from build123d import *

# Parameters (mm, degrees)
F2_SIZE2 = 1.8330871047
F2_SIZE  = 3.175
F3_R     = 0.762
F4_R     = 0.254
F5_SIZE  = 0.508
F6_R     = 2.0447
F7_DEPTH = 25.4


with BuildPart() as f1:
    # F0 (on Front) → F1 (revolve)
    with BuildSketch(Plane.XZ):
        Polygon((11.1125, 23.68296), (11.1125, 31.75), (0, 31.75), (0, 17.3101), (33.3375, 17.3101), (33.3375, 23.68296), (25.5905, 23.68296), (25.5905, 19.09445), (18.3261, 19.09445), (18.3261, 23.68296), align=None)
    revolve(axis=Axis((23.780265148, 0, 0), (1, 0, 0)))

    # F2
    f2_edges = [f1.edges().sort_by_distance(p)[0] for p in [
        (33.3375, 0, -23.68296),
    ]]
    f2_side = f1.faces().sort_by_distance((29.464, 0, -23.68296))[0]
    chamfer(f2_edges, length=F2_SIZE, length2=F2_SIZE2, reference=f2_side)

    # F3
    f3_edges = [f1.edges().sort_by_distance(p)[0] for p in [
        (18.3261, 0, -19.09445),
        (25.5905, 0, -19.09445),
    ]]
    fillet(f3_edges, radius=F3_R)

    # F4
    f4_edges = [f1.edges().sort_by_distance(p)[0] for p in [
        (11.1125, 0, -23.68296),
    ]]
    fillet(f4_edges, radius=F4_R)

    # F5
    f5_edges = [f1.edges().sort_by_distance(p)[0] for p in [
        (11.1125, 0, -31.75),
        (0, 0, -31.75),
    ]]
    chamfer(f5_edges, length=F5_SIZE)

    # F6 (on Right) → F7 (cut)
    with BuildSketch(Plane.YZ):
        with Locations((0, 26.9875)):
            Circle(F6_R)
        with Locations((23.3718605846, -13.49375)):
            Circle(F6_R)
        with Locations((-23.3718605846, -13.49375)):
            Circle(F6_R)
    extrude(amount=F7_DEPTH, mode=Mode.SUBTRACT)


solid = f1.part
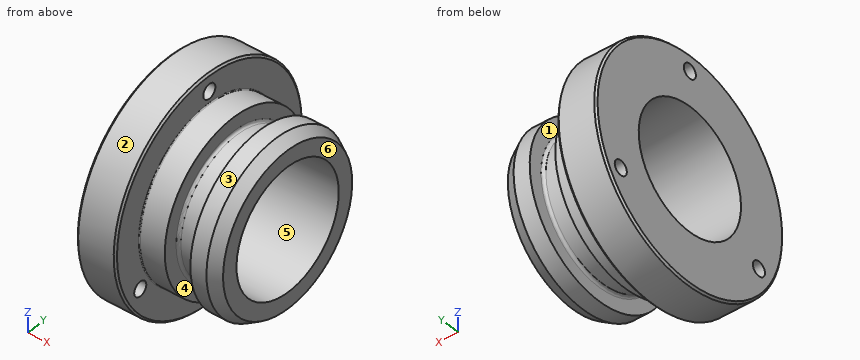
Input: part model. Units: mm. Frame: model coordinates. Face numbers are marked on the shaded views. A direction names the side the tool comes from. Coordinates: 2 decimals unless noted, no trailing zeros. Write each loop counter-clockwise with the first axis right and the second up, starting at its lowest first coordinate (ties: lowest second). Pieces come first, ordered by that corner, then holes. Notation, with made-up numbers: M 22.25,84.5 L 37.25,84.5 A18 cw 37.25,94.5 Z; hole C 30.25,-31 d10. An arc over 180 degrees is marked long. Answer as a JSON object with one key per item and string values. Group by question number.
(1) Mould query, pull axis X, two halves, no side actions, for the marked faces 4, 5 and 6. Classes: pulls with the +X half, pulls with the -X half, needs draft (parallel to the pull), parting line crosses it, or undercut.
(2) Set-up query: the marked faces 1, 2 and 3. Return all of +Z, -Z, +X, -X, +Y, -Y with unobstructed straight access to the full face (end or side cutting, diameter ignored); none if empty.
(3) Section B-B on y = 0. Give the number of separate pieces and of enclosed holes in the cut face, plus the area to 3 significant figures.
(4) Section C-C on x = 26.5. Output: boundary loops of the cut face in (y, z), plus the area to 3 significant figures.
(5) Ray query, line 1 along Z through (x, y) = (3, 0); line 2 along X through (y, z) = (21, 1); line 3 along Y through (x, z) = (14, 0). Return the intervals inside material, ascending. Write a range as [from, to].
(6) Contact query for flat-ended pins moving along their axis: P1, Ø3.5, axis at y = 0, z = 26.99, coming from the -X side; P2, Ø8, axis at x = 15.5, y = -19, coming from the -Z side; P3, Ø8, axis at y = -13.5, z = -7, coming from the +X side; P4, Ø8, axis at x = 19, y = 23, coming from the +Z side. Output: stop coordinate, or through.
(7) Section D-D on x = 3. Output: boundary loops of the cut face in (y, z).
Result set:
{
 "1": {"face 4": "undercut", "face 5": "needs draft", "face 6": "pulls with the +X half"},
 "2": {"face 1": "none", "face 2": "+X, -X", "face 3": "+X"},
 "3": {"separate pieces": "3", "enclosed holes": "0", "area": "486 mm2"},
 "4": {"outline": "C 0,0 d47.37; hole C 0,0 d34.62", "area": "821 mm2"},
 "5": {"line 1": "z = [-31.75, -17.31], [17.31, 24.94], [29.03, 31.75]", "line 2": "x = [0, 18.33], [25.59, 33.34]", "line 3": "y = [-23.68, -17.31], [17.31, 23.68]"},
 "6": {"P1": "passes through", "P2": "stops at z = -18.33", "P3": "stops at x = 33.34", "P4": "stops at z = 14.06"},
 "7": {"outline": "C 0,0 d63.5; hole C -23.37,-13.49 d4.09; hole C 0,0 d34.62; hole C 0,26.99 d4.09; hole C 23.37,-13.49 d4.09"}
}
